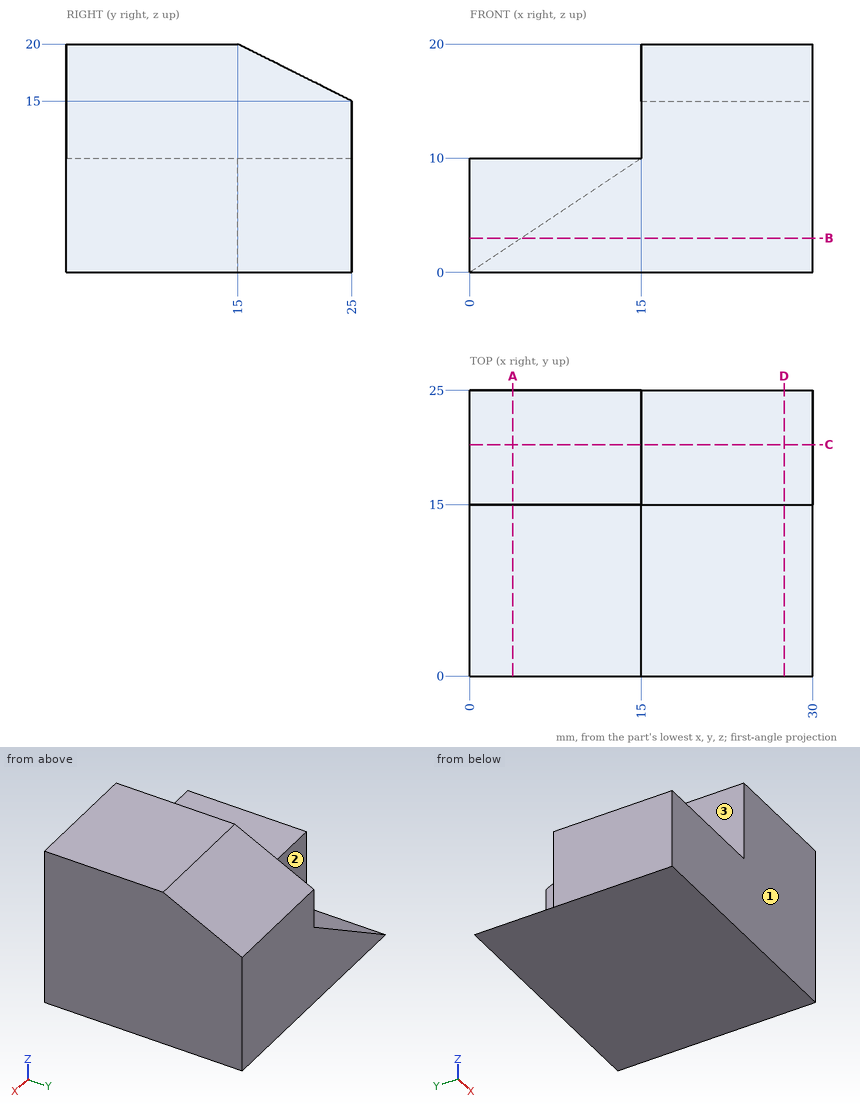
Can you work these out from the drawing? Everything is in mm from the part's minimum corner. A direction names the side the tool comes from. Give positions to 0.01 mm unless a question says otherwise; leave off trailing zeros. Loops run counter-clockwise (first coordinate to the right, second up) from the corner with the lowest first, then second, coordinate; pieces in that order, holes last. Notation, with made-up numbers: (19, 35.25) - (31, 35.25) arc R24 cw to (31, 69.25) - close; hole circle Ø7 at (19, 16). An arc over 180 degrees is marked (long way). Answer as a JSON object with one key per item and string values.
Q1. Imagine slicing it at B-B on z = 3. Write out the boundary of the cut face in (x, y).
Geometry says:
{"outline": "(0, 0) - (30, 0) - (30, 25) - (4.5, 25) - (4.5, 15) - (0, 15) - close"}
Q2. If I drill on L1, parallel to X at y = 1.25, z = 12; L2, parallel to Z at x = 6.25, y = 14.5; L3, parallel to X at y = 22, z = 3.75 (3 decimals), over which ranges is the centre line in solid material (lowest first)?
Geometry says:
{"L1": "15 to 30", "L2": "0 to 10", "L3": "5.625 to 30"}
Q3. Imagine slicing it at A-A on x = 3.75. Write out the boundary of the cut face in (y, z), plus the area to 3 significant figures.
Geometry says:
{"outline": "(0, 0) - (25, 0) - (25, 2.5) - (15, 2.5) - (15, 10) - (0, 10) - close", "area": "175 mm²"}
Q4. Imagine slicing it at D-D on x = 27.5. Write out the boundary of the cut face in (y, z), plus the area to 3 significant figures.
Geometry says:
{"outline": "(0, 0) - (25, 0) - (25, 15) - (15, 20) - (0, 20) - close", "area": "475 mm²"}
Q5. Will these pins go through, and if not, where does the flat tip stop? P1, Ø3, axis at x = 4, z = 6, coming from the +Y side; P2, Ø4.5, axis at x = 6, y = 10.5, coming from the +Z side; P3, Ø6, axis at y = 18, z = 15, coming from the -X side.
Geometry says:
{"P1": "y = 15", "P2": "z = 10", "P3": "x = 15"}
Q6. Which directions (+Z, -Z, +X, -X, +Y, -Y) give clear straight access to the entire face, cutting with the end or side of a thin tool? Please do the marked faces 1, 2 and 3.
Geometry says:
{"face 1": "+Z, -Z, +X, -X, -Y", "face 2": "+Z, -X, +Y", "face 3": "+Z, -X, +Y, -Y"}
Q7. Imagine slicing it at C-C on y = 20.25. Write out the boundary of the cut face in (x, z) (3 decimals), plus the area to 3 significant figures.
Geometry says:
{"outline": "(0, 0) - (30, 0) - (30, 17.375) - (15, 17.375) - (15, 10) - close", "area": "336 mm²"}
